Can you work these out from the model? Positions are in its coordinate system, mm. Give positions to 0.01 mm unless a question says otherwise; leave off trailing zeros. Order: outer loops, then holes, each group sorted by start corner. A loop starts at its lowest first (then second) coordinate and runs counter-clockwise, first axis right, second up.
Item 1: I want a section at D-D, the plane z = 2.9. Count the separate pieces of the cut face and the enclosed holes in it, then the cut area to 3 significant figures.
Item 2: I want a section at C-C, the plane x = 8.5. Write out the boundary of the cut face in (y, z).
Item 3: I want a section at B-B, the plane x = 45. Write out the boundary of the cut face in (y, z), then the cut area to 3 significant figures.
Item 4: I want a section at A-A, the plane y = 77. Write out the boundary of the cut face in (x, z), then the cut area to 3 significant figures.
Item 5: I'm going to push flat-ended pins straight in: pin 1 Ø2 at (y, z) = (70, 2.5) entering from -X; pin 2 Ø0.5 at (y, z) = (72, 3.5) entering from -X; pin 3 Ø1.5 at (x, z) = (2, 3.5) entering from +Y. Where does each tip first touch, or does it pass through?
Item 6: If I drill on line 1 along Y through (x, z) = (15, 3.95); line 2 along X through (y, z) = (67.5, 4.2); line 3 along Y through (x, z) = (28.5, 1.95), over which ranges is the centre line in solid material (lowest first)?
```python
from build123d import *

# Parameters (mm, degrees)
ESQUISSE1_R        = 2
BOSS_EXTRU_1_DEPTH = 5
CONG_1_R           = 10


with BuildPart() as part:
    # Esquisse1 → Boss.-Extru.1 (new body)
    with BuildSketch(Plane.XY):
        Polygon((0, 80), (0, 100), (60, 100), (60, 60), (40, 0), (0, 0), (0, 60), (-5, 60), (-5, 65), (0, 65), (0, 68.5), (3, 68.5), (3, 67.4), (5.3, 67.4), (5.3, 68.5), (10, 68.5), (10, 71.5), (5.3, 71.5), (5.3, 72.6), (3, 72.6), (3, 71.5), (0, 71.5), (0, 75), (-5, 75), (-5, 80), align=None)
        with Locations((15, 77)):
            Circle(ESQUISSE1_R, mode=Mode.SUBTRACT)
        with Locations((30, 77)):
            Circle(ESQUISSE1_R, mode=Mode.SUBTRACT)
        with Locations((45, 77)):
            Circle(ESQUISSE1_R, mode=Mode.SUBTRACT)
        with Locations((45, 63)):
            Circle(ESQUISSE1_R, mode=Mode.SUBTRACT)
        with Locations((30, 63)):
            Circle(ESQUISSE1_R, mode=Mode.SUBTRACT)
        with Locations((15, 63)):
            Circle(ESQUISSE1_R, mode=Mode.SUBTRACT)
    extrude(amount=BOSS_EXTRU_1_DEPTH)

    # Congé1
    cong_1_edges = [part.edges().sort_by_distance(p)[0] for p in [
        (0, 100, 2.5),
        (60, 100, 2.5),
        (60, 60, 2.5),
        (40, 0, 2.5),
        (0, 0, 2.5),
    ]]
    fillet(cong_1_edges, radius=CONG_1_R)


solid = part.part
```
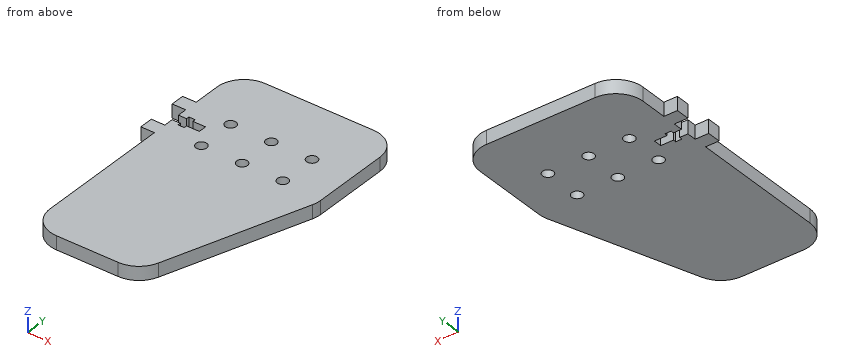
Results list:
1. separate pieces: 1
1. enclosed holes: 6
1. area: 5,270 mm2
2. outline: (0.11, 0) - (68.5, 0) - (68.5, 5) - (0.11, 5) - close; (71.5, 0) - (99.89, 0) - (99.89, 5) - (71.5, 5) - close
3. outline: (15, 0) - (61, 0) - (61, 5) - (15, 5) - close; (65, 0) - (75, 0) - (75, 5) - (65, 5) - close; (79, 0) - (100, 0) - (100, 5) - (79, 5) - close
3. area: 385 mm2
4. outline: (-5, 0) - (13, 0) - (13, 5) - (-5, 5) - close; (17, 0) - (28, 0) - (28, 5) - (17, 5) - close; (32, 0) - (43, 0) - (43, 5) - (32, 5) - close; (47, 0) - (60, 0) - (60, 5) - (47, 5) - close
4. area: 265 mm2
5. pin 1: stops at x = 10
5. pin 2: stops at x = 0
5. pin 3: stops at y = 96.89
6. line 1: y = 0 to 61, 65 to 75, 79 to 100
6. line 2: x = 0 to 3, 5.3 to 60
6. line 3: y = 0 to 61.68, 64.32 to 75.68, 78.32 to 100
